from build123d import *

# Parameters (mm, degrees)
CROQUIS1_R              = 57.226702921
CROQUIS1_R_2            = 7.277968804
CROQUIS1_R_3            = 9.940183118
CROQUIS1_R_4            = 20.796607535
SALIENTE_EXTRUIR1_DEPTH = 10
CROQUIS2_R              = 23.842859528
SALIENTE_EXTRUIR2_DEPTH = 10
CROQUIS3_R              = 8.254589986
CORTAR_EXTRUIR1_DEPTH   = 10


with BuildPart() as part:
    # Croquis1 → Saliente-Extruir1 (new body)
    with BuildSketch(Plane.XY):
        Circle(CROQUIS1_R)
        with Locations((-4.741989664, 34.759410431)):
            Circle(CROQUIS1_R_2, mode=Mode.SUBTRACT)
        with Locations((-4.741989664, -33.045918367)):
            Circle(CROQUIS1_R_3, mode=Mode.SUBTRACT)
        with Locations((29.772636186, 4.89569161)):
            Circle(CROQUIS1_R_4, mode=Mode.SUBTRACT)
    extrude(amount=SALIENTE_EXTRUIR1_DEPTH)

    # Croquis2 → Saliente-Extruir2 (add)
    with BuildSketch(Plane.XY.offset(10)):
        with Locations((-57.226702921, 0)):
            Circle(CROQUIS2_R)
    extrude(amount=SALIENTE_EXTRUIR2_DEPTH)

    # Croquis3 → Cortar-Extruir1 (cut)
    with BuildSketch(Plane.XY.offset(10)):
        with Locations((-17.135779728, 9.968610226)):
            Circle(CROQUIS3_R)
    extrude(amount=-CORTAR_EXTRUIR1_DEPTH, mode=Mode.SUBTRACT)


solid = part.part
Read the model definition and answer for the solid it produces. Units are mm, in the model's axes. Coordinates: 2 decimals unless noted, no trailing zeros. Order: outer loops, then holes, each group sorted by start corner. A loop starts at its lowest first (then second) coordinate and runs counter-clockwise, first axis right, second up. Notation, with made-up numbers: M 36.5,-9 L 75.5,-9 A26 ccw 75.5,13 Z; hole C -31,-13.5 d10. An arc over 180 degrees is marked long. Put each result on its own line as item: value. Start each with the question number.
Item 1: Section B-B, the plane x = 0 is taken. Determine the outline of the cut face in (y, z), plus the area to 3 significant figures.
Item 2: Section A-A, the plane y = 20.5 is taken. Determine the outline of the cut face in (x, z).
Item 3: Section D-D, the plane x = -49.5 is taken. Determine the outline of the cut face in (y, z).
Item 4: Consider probe 1 along Z at (x, y) = (-26, 48); probe 2 along X at (y, z) = (8, 7.25); probe 3 along Y at (x, z) = (-24.5, 7). Determine where each line is inside the solid, lowest interval first. Write a range as [from, to].
Item 5: Given pin 1 Ø13 at (x, y) = (-4.74, 34.76) entering from +Z; pin 2 Ø2 at (y, z) = (21.5, 11.5) entering from +X; pin 3 Ø3 at (y, z) = (-31, 3.5) entering from -X; pin 4 Ø8 at (x, z) = (-30.5, 6.5) entering from -Y, each flat-ended and moving along its own axis, determine where each tip first touches the part or whether it passes through.
Item 6: Section C-C, the plane x = 24 is taken. Determine the outline of the cut face in (y, z).
Item 7: The mould has two halves that part along X. Classify faces 1 (the face through (-34.485, 7.162, 14.93)), 2 (the face through (13.3, -7.8, 4.9)), 3 (the face through (-1, 1, 0)): +X half, -X half, draft (parallel to the pull), parting line (faces both ways), or undercut.
Computed:
1. outline: M -57.23,0 L -41.78,0 L -41.78,10 L -57.23,10 Z; M -24.31,0 L 29.24,0 L 29.24,10 L -24.31,10 Z; M 40.28,0 L 57.23,0 L 57.23,10 L 40.28,10 Z
1. area: 859 mm2
2. outline: M -69.4,10 L -53.43,10 L -53.43,0 L 16.02,0 L 16.02,10 L -45.05,10 L -45.05,20 L -69.4,20 Z; M 43.52,0 L 53.43,0 L 53.43,10 L 43.52,10 Z
3. outline: M -28.72,0 L 28.72,0 L 28.72,10 L 22.56,10 L 22.56,20 L -22.56,20 L -22.56,10 L -28.72,10 Z
4. probe 1: z = [0, 10]
4. probe 2: x = [-56.66, -25.15], [-9.12, 9.21], [50.34, 56.66]
4. probe 3: y = [-51.72, 6.24], [13.7, 51.72]
5. pin 1: passes through
5. pin 2: stops at x = -45.05
5. pin 3: stops at x = -49.04
5. pin 4: stops at y = -50.72
6. outline: M -51.95,0 L -15.08,0 L -15.08,10 L -51.95,10 Z; M 24.88,0 L 51.95,0 L 51.95,10 L 24.88,10 Z
7. face 1: parting line
7. face 2: undercut
7. face 3: draft
